The listing builds one solid part. Answer for the finished solid, in the listing's coordinates (mm). A direction names the side the tool comes from. Coordinates: 2 decimals unless noted, no trailing zeros. Order: outer loops, then holes, each group sorted by start corner. A loop starts at its lowest first (then second) coordinate and runs counter-clockwise, first axis right, second up. Notation, with made-up numbers: M 47,-25.5 L 69,-25.5 A29 cw 69,5.5 Z; hole C -6.5,2 d4. An arc over 180 degrees is marked long. One line per item, written item: value. Start each with the question number.
Q1. This flat-tipped pin is pushed along its axis until it touches: pin 1 Ø4.5 at (x, y) = (-18.38, -18.38) entering from -Z. Where does it stop, or does it pass through?
Q2. Determine the mould class of faces 1 (the cylindrical face through (47.973, 51.859, 4.93)), 2 (the cylindrical face through (-62.15, -61.99, 4.93)), 3 (the cylindrical face through (62.15, 61.99, 4.93)) for opening direction X: pulls with the +X half, pulls with the -X half, needs draft (parallel to the pull), parting line crosses it, or undercut.
Q3. The part is cut by section C-C on x = 37.5. Give the vertices of the cut face in (y, z), then the cut area to 3 significant figures.
Q4. The part is cut by section A-A on y = 0. Give the vertices of the cut face in (x, z), then the cut area to 3 significant figures.
Q5. Straight lines are drawn through the part: line 1 along Y through (x, z) = (0, 2); line 2 along X through (y, z) = (7, 1) (3 decimals); line 3 along Y through (x, z) = (-1.5, 9). For each, find the intervals that lie inside material, in ascending order. Write a range as [from, to].
Q6. The part is cut by section D-D on z = 7.75. Give the number of separate pieces and of enclosed holes in the cut face, then the cut area to 3 significant figures.
Q7. For faces 4 (the flat face through (35, 0, 5)), 5 (the flat face through (1, 65, 5)), determine the directions among +Z, -Z, +X, -X, +Y, -Y from which every point of the face is accessible in a straight line to the end or side of a thin tool.
```python
from build123d import *

# Parameters (mm, degrees)
F0_R     = 2.75
F0_R_2   = 20
F1_DEPTH = 10


with BuildPart() as f1:
    # F0 (on Top) → F1 (new body)
    with BuildSketch(Plane.XY):
        with BuildLine():
            Line((-55, -65), (55, -65))
            ThreePointArc((55, -65), (62.071068, -62.071068), (65, -55))
            Line((65, -55), (65, 55))
            ThreePointArc((65, 55), (62.071068, 62.071068), (55, 65))
            Line((55, 65), (-55, 65))
            ThreePointArc((-55, 65), (-62.071068, 62.071068), (-65, 55))
            Line((-65, 55), (-65, -55))
            ThreePointArc((-65, -55), (-62.071068, -62.071068), (-55, -65))
        make_face()
        with Locations((-50, -50)):
            Circle(F0_R, mode=Mode.SUBTRACT)
        with BuildLine():
            Line((-22.580764, -35), (22.419236, -35))
            ThreePointArc((22.419236, -35), (29.919671, -42.420101), (22.580764, -50))
            Line((22.580764, -50), (-22.419236, -50))
            ThreePointArc((-22.419236, -50), (-29.919671, -42.579899), (-22.580764, -35))
        make_face(mode=Mode.SUBTRACT)
        with BuildLine():
            Line((-35, 22.580764), (-35, -22.419236))
            ThreePointArc((-35, -22.419236), (-42.418362, -30.081198), (-50, -22.580764))
            Line((-50, -22.580764), (-50, 22.419236))
            ThreePointArc((-50, 22.419236), (-42.579899, 29.919671), (-35, 22.580764))
        make_face(mode=Mode.SUBTRACT)
        with Locations((-18.384776, -18.384776)):
            Circle(F0_R, mode=Mode.SUBTRACT)
        with Locations((50, -50)):
            Circle(F0_R, mode=Mode.SUBTRACT)
        with Locations((18.384776, -18.384776)):
            Circle(F0_R, mode=Mode.SUBTRACT)
        with Locations((-18.384776, 18.384776)):
            Circle(F0_R, mode=Mode.SUBTRACT)
        with Locations((-50, 50)):
            Circle(F0_R, mode=Mode.SUBTRACT)
        Circle(F0_R_2, mode=Mode.SUBTRACT)
        with Locations((18.384776, 18.384776)):
            Circle(F0_R, mode=Mode.SUBTRACT)
        with BuildLine():
            Line((50, 22.419236), (50, -22.580764))
            ThreePointArc((50, -22.580764), (42.420101, -29.919671), (35, -22.419236))
            Line((35, -22.419236), (35, 22.580764))
            ThreePointArc((35, 22.580764), (42.581638, 30.081198), (50, 22.419236))
        make_face(mode=Mode.SUBTRACT)
        with BuildLine():
            ThreePointArc((22.580764, 50), (30.081198, 42.418362), (22.419236, 35))
            Line((22.419236, 35), (-22.580764, 35))
            ThreePointArc((-22.580764, 35), (-29.919671, 42.579899), (-22.419236, 50))
            Line((-22.419236, 50), (22.580764, 50))
        make_face(mode=Mode.SUBTRACT)
        with Locations((50, 50)):
            Circle(F0_R, mode=Mode.SUBTRACT)
    extrude(amount=F1_DEPTH)


solid = f1.part
```
Output:
1. pin 1: passes through
2. face 1: undercut
2. face 2: pulls with the -X half
2. face 3: pulls with the +X half
3. outline: M -65,0 L -28.01,0 L -28.01,10 L -65,10 Z; M 28.17,0 L 65,0 L 65,10 L 28.17,10 Z
3. area: 738 mm^2
4. outline: M -65,0 L -50,0 L -50,10 L -65,10 Z; M -35,0 L -20,0 L -20,10 L -35,10 Z; M 20,0 L 35,0 L 35,10 L 20,10 Z; M 50,0 L 65,0 L 65,10 L 50,10 Z
4. area: 600 mm^2
5. line 1: y = [-65, -50], [-35, -20], [20, 35], [50, 65]
5. line 2: x = [-65, -50], [-35, -18.735], [18.735, 35], [50, 65]
5. line 3: y = [-65, -50], [-35, -19.94], [19.94, 35], [50, 65]
6. separate pieces: 1
6. enclosed holes: 13
6. area: 12,000 mm^2
7. face 4: +Z, -Z
7. face 5: +Z, -Z, +X, -X, +Y
